from build123d import *

# Parameters (mm, degrees)
SKETCH1_W               = 70
SKETCH1_H               = 60
BOSS_EXTRUDE2_DEPTH     = 8
CUT_EXTRUDE3_DEPTH      = 37
CUT_EXTRUDE3_DEPTH_BACK = 30
SKETCH1_5_R             = 2.75
CUT_EXTRUDE4_DEPTH      = 30
CUT_EXTRUDE4_DEPTH_BACK = 30
SKETCH1_7_R             = 2.75
CUT_EXTRUDE5_DEPTH      = 42
CUT_EXTRUDE5_DEPTH_BACK = 88
SKETCH1_8_R             = 5
CUT_EXTRUDE6_DEPTH      = 42
SKETCH1_9_R             = 5
CUT_EXTRUDE7_DEPTH      = 5.4
SKETCH1_10_R            = 5
CUT_EXTRUDE8_DEPTH      = 5.4


with BuildPart() as part:
    # Sketch1 → Boss-Extrude2 (new body)
    with BuildSketch(Plane.XY):
        with Locations((-22.732855119, 15.168432036)):
            Rectangle(SKETCH1_W, SKETCH1_H)
    extrude(amount=BOSS_EXTRUDE2_DEPTH)

    # Sketch1_5 → Cut-Extrude3 (cut, two sides: drawn at the far end of the back side and taken through both)
    with BuildSketch(Plane.XY.offset(-CUT_EXTRUDE3_DEPTH_BACK)):
        with Locations(Location((-47.732855119, -8.831567964, 0), (0, 0, 180))):
            Circle(SKETCH1_5_R)
    extrude(amount=CUT_EXTRUDE3_DEPTH + CUT_EXTRUDE3_DEPTH_BACK, mode=Mode.SUBTRACT)

    # Sketch1_7 → Cut-Extrude4 (cut, two sides: drawn at the far end of the back side and taken through both)
    with BuildSketch(Plane.XY.offset(-CUT_EXTRUDE4_DEPTH_BACK)):
        with Locations(Location((2.267144881, -8.831567964, 0), (0, 0, 180))):
            Circle(SKETCH1_7_R)
    extrude(amount=CUT_EXTRUDE4_DEPTH + CUT_EXTRUDE4_DEPTH_BACK, mode=Mode.SUBTRACT)

    # Sketch1_8 → Cut-Extrude5 (cut, two sides: drawn at the far end of the back side and taken through both)
    with BuildSketch(Plane.XY.offset(-CUT_EXTRUDE5_DEPTH_BACK)):
        with Locations(Location((-22.732855119, 33.168432036, 0), (0, 0, 180))):
            Circle(SKETCH1_8_R)
    extrude(amount=CUT_EXTRUDE5_DEPTH + CUT_EXTRUDE5_DEPTH_BACK, mode=Mode.SUBTRACT)

    # Sketch3 → Cut-Extrude6 (cut)
    with BuildSketch(Plane.XY.offset(8)):
        Polygon((-48.232855119, 45.168432036), (-57.732855119, 38.168432036), (-57.732855119, 45.168432036), align=None)
        Polygon((2.767144881, 45.168432036), (12.267144881, 38.168432036), (12.267144881, 45.168432036), align=None)
    extrude(amount=-CUT_EXTRUDE6_DEPTH, mode=Mode.SUBTRACT)

    # Sketch1_9 → Cut-Extrude7 (cut)
    with BuildSketch(Plane.XY):
        with Locations(Location((-47.732855119, -8.831567964, 0), (0, 0, 180))):
            Circle(SKETCH1_9_R)
    extrude(amount=CUT_EXTRUDE7_DEPTH, mode=Mode.SUBTRACT)

    # Sketch1_10 → Cut-Extrude8 (cut)
    with BuildSketch(Plane.XY):
        with Locations(Location((2.267144881, -8.831567964, 0), (0, 0, 180))):
            Circle(SKETCH1_10_R)
    extrude(amount=CUT_EXTRUDE8_DEPTH, mode=Mode.SUBTRACT)


solid = part.part
Model file for the job. Use its own axes, mm. A direction names the side the tool comes from. Give positions to 0.01 mm unless a question says otherwise; leave off trailing zeros. Loops run counter-clockwise (first coordinate to the right, second up) from the corner with the lowest first, then second, coordinate; pieces in that order, holes last.
1) Pull direction Y, two halves, no side cores. Call faces 1 (the flat face through (-23, -14.832, 4)), 2 (the flat face through (-23, 16, 8)), 3 (the flat face through (7.45, 41.72, 4.06)), 4 (the cylindrical face through (-0.356, -9.658, 6.682)): +Y half, -Y half, draft (parallel to the pull), parting line (faces both ways), or undercut.
2) Tool access for faces 5 (the flat face through (-57.733, 11, 4)), 6 (the flat face through (-50, -7, 5.4)): list every direction of +Z, -Z, +X, -X, +Y, -Y with a clear straight run to the whole face (end or side of a thin tool).
3) Saw through at A-A (x = -25.5). Write the cut outline in (y, z).
4) Flat gauge pins, fed straight in: pin 1 Ø8 at (x, y) = (2.27, -8.83) entering from -Z; pin 2 Ø3 at (x, y) = (1.5, -8) entering from -Z. Where does each tip first touch, or does it go through?
5) Wall check: line 1 (Y direction, x = -48, z = 4.25); line 2 (Y direction, x = -25.5, z = 3); line 3 (Z direction, x = 1.5, y = -6). Give the ranges that are in metal, low to high.
6) Saw through at D-D (y = 39). Write the cut outline in (x, z), plus the area to 3 significant figures.
7) Saw through at B-B (y = 29.5). Write the cut outline in (x, z).
8) Saw through at C-C (z = 6.25). Write the cut outline in (x, y).
Answer block:
1. face 1: -Y half
1. face 2: draft
1. face 3: +Y half
1. face 4: undercut
2. face 5: +Z, -Z, -X, +Y, -Y
2. face 6: -Z
3. outline: (-14.83, 0) - (29, 0) - (29, 8) - (-14.83, 8) - close; (37.33, 0) - (45.17, 0) - (45.17, 8) - (37.33, 8) - close
4. pin 1: stops at z = 5.4
4. pin 2: passes through
5. line 1: y = -14.83 to -13.82, -3.84 to 45.17
5. line 2: y = -14.83 to 29, 37.33 to 45.17
5. line 3: z = 5.4 to 8
6. outline: (-56.6, 0) - (11.14, 0) - (11.14, 8) - (-56.6, 8) - close
6. area: 542 mm2
7. outline: (-57.73, 0) - (-26.13, 0) - (-26.13, 8) - (-57.73, 8) - close; (-19.34, 0) - (12.27, 0) - (12.27, 8) - (-19.34, 8) - close
8. outline: (-57.73, -14.83) - (12.27, -14.83) - (12.27, 38.17) - (2.77, 45.17) - (-48.23, 45.17) - (-57.73, 38.17) - close; hole circle Ø5.5 at (-47.73, -8.83); hole circle Ø10 at (-22.73, 33.17); hole circle Ø5.5 at (2.27, -8.83)
